The listing builds one solid part. Answer for the finished solid, in the listing's coordinates (mm). Coordinates: 2 decimals unless noted, no trailing zeros. Order: outer loops, then holes, each group sorted by start corner. A loop starts at its lowest first (then second) coordinate and runs counter-clockwise, first axis right, second up. Notation, with made-up numbers: (17, -2.75) - (38, -2.75) arc R16 ccw to (38, 3.25) - close; hole circle Ø6 at (71.5, 83). An arc over 180 degrees is marked (long way). One line per item, written item: value. Start each with the question number.
```python
from build123d import *

# Parameters (mm, degrees)
BOSS_EXTRUDE1_DEPTH = 22.225
SKETCH2_R           = 3.175
CUT_EXTRUDE1_DEPTH  = 22.225


with BuildPart() as part:
    # Sketch1 → Boss-Extrude1 (new body)
    with BuildSketch(Plane(origin=(0, 0, 0), x_dir=(0, 0, -1), z_dir=(1, 0, 0))):
        Polygon((0, -5.55625), (0, 5.55625), (-3.207902433, 5.55625), (-6.415804866, 0), (-3.207902433, -5.55625), align=None)
        Polygon((3.207902433, 5.55625), (0, 5.55625), (0, -5.55625), (3.207902433, -5.55625), (6.415804866, 0), align=None)
    extrude(amount=BOSS_EXTRUDE1_DEPTH)

    # Sketch2 → Cut-Extrude1 (cut)
    with BuildSketch(Plane.ZY):
        Circle(SKETCH2_R)
    extrude(amount=-CUT_EXTRUDE1_DEPTH, mode=Mode.SUBTRACT)


solid = part.part
```
(1) The part is cut by section C-C on y = 1.5. Determine the outline of the cut face in (x, z) (3 decimals), plus the area to 3 significant figures.
(2) For a pull along Z with two mould halves and no side action, classify faces 1 (the face through (11, -2.8, -4.8)), 2 (the face through (10.957, -2.739, 4.834)), 3 (the face through (22.225, 3, -3)), 4 (the face through (10.96, -3.1, -0.69)) as pulls with the +Z half, pulls with the -Z half, needs draft (parallel to the pull), parting line crosses it, or undercut.
(3) Consider probe 1 along Y at (x, z) = (9.5, 0) (3 decimals); probe 2 along Y at (x, z) = (19, -2.5); probe 3 along Z at (x, y) = (14.5, 2.5). Determine where each line is inside the solid, lowest interval first.
(4) The part is cut by section B-B on z = 0. Determine the outline of the cut face in (x, y) (3 decimals), plus the area to 3 significant figures.
(5) The part is cut by section A-A on x = 18. Determine the outline of the cut face in (y, z) (3 decimals), plus the area to 3 significant figures.
(6) The part is cut by section D-D on z = -5.25. Determine the outline of the cut face in (x, y) (3 decimals).
(7) A flat-ended cylindrical pin translates along its axis: pin 1 Ø5 at (y, z) = (0, 0) entering from +X. Find the tip coordinate at first contact, or state that the pin passes through.
Completed:
1. outline: (0, -5.55) - (22.225, -5.55) - (22.225, -2.798) - (0, -2.798) - close; (0, 2.798) - (22.225, 2.798) - (22.225, 5.55) - (0, 5.55) - close
1. area: 122 mm2
2. face 1: pulls with the -Z half
2. face 2: pulls with the +Z half
2. face 3: needs draft
2. face 4: undercut
3. probe 1: y = -5.556 to -3.175, 3.175 to 5.556
3. probe 2: y = -5.56 to -1.96, 1.96 to 5.56
3. probe 3: z = -4.97 to -1.96, 1.96 to 4.97
4. outline: (0, -5.556) - (22.225, -5.556) - (22.225, -3.175) - (0, -3.175) - close; (0, 3.175) - (22.225, 3.175) - (22.225, 5.556) - (0, 5.556) - close
4. area: 106 mm2
5. outline: (-5.556, -3.208) - (0, -6.416) - (5.556, -3.208) - (5.556, 3.208) - (0, 6.416) - (-5.556, 3.208) - close; hole circle Ø6.35 at (0, 0)
5. area: 75.3 mm2
6. outline: (0, -2.019) - (22.225, -2.019) - (22.225, 2.019) - (0, 2.019) - close
7. pin 1: passes through
